Model file for the job. Use its own axes, mm. A direction names the side the tool comes from. Give positions to 0.01 mm unless a question says otherwise; leave off trailing zeros. Write each loop counter-clockwise with the first axis right and the second up, starting at its lowest first coordinate (ties: lowest second). Pieces come first, ordered by that corner, then holes. Notation, with made-up numbers: M 75,48.5 L 131,48.5 A18 cw 131,71.5 Z; hole C -15.75,15.25 d5. An arc over 180 degrees is marked long. Answer as a JSON object with one key per item and string values. Group by question number.
```python
from build123d import *

# Parameters (mm, degrees)
SKETCH_1_W          = 15
SKETCH_1_H          = 15
EXTRUDE_1_DEPTH     = 100
SKETCH_2_W          = 45
SKETCH_2_H          = 15
EXTRUDE_2_DEPTH     = 10
SKETCH_3_R          = 2.5
CUT_EXTRUDE_1_DEPTH = 20
SKETCH_5_W          = 45
SKETCH_5_H          = 19.472765692
EXTRUDE_3_DEPTH     = 10
SKETCH_6_R          = 2.5
CUT_EXTRUDE_2_DEPTH = 103.961386699


with BuildPart() as part:
    # 草图1 → 凸台-拉伸1 (new body)
    with BuildSketch(Plane.XY):
        Rectangle(SKETCH_1_W, SKETCH_1_H)
    extrude(amount=EXTRUDE_1_DEPTH)

    # 草图2 → 凸台-拉伸2 (add)
    with BuildSketch(Plane.XY.offset(100)):
        Rectangle(SKETCH_2_W, SKETCH_2_H)
    extrude(amount=-EXTRUDE_2_DEPTH)

    # 草图3 → 切除-拉伸1 (cut)
    with BuildSketch(Plane.XY.offset(100)):
        with Locations((-16.5, 0)):
            Circle(SKETCH_3_R)
        with Locations((16.5, 0)):
            Circle(SKETCH_3_R)
    extrude(amount=-CUT_EXTRUDE_1_DEPTH, mode=Mode.SUBTRACT)

    # 草图5 → 凸台-拉伸3 (add)
    with BuildSketch(Plane(origin=(0, 0, 0), x_dir=(-1, 0, 0), z_dir=(0, 0, -1))):
        Rectangle(SKETCH_5_W, SKETCH_5_H)
    extrude(amount=-EXTRUDE_3_DEPTH)

    # 草图6 → 切除-拉伸2 (cut, through all)
    with BuildSketch(Plane(origin=(0, 0, 0), x_dir=(-1, 0, 0), z_dir=(0, 0, -1))):
        with Locations(Location((-16.5, 0, 0), (0, 0, 180))):
            Circle(SKETCH_6_R)
        with Locations(Location((16.5, 0, 0), (0, 0, 180))):
            Circle(SKETCH_6_R)
    extrude(amount=-CUT_EXTRUDE_2_DEPTH, mode=Mode.SUBTRACT)


solid = part.part
```
Q1. Slice it at B-B, the plane x = 16.5. Write the cut outline in (y, z).
Q2. Slice it at D-D, the plane y = -6.25. Write the cut outline in (x, z).
Q3. 3-axis set-ups, long thin cutter, end or side, ignore diameter. For faces 4 (the flat face through (7.5, 0, 49)), 5 (the flat face through (0, -7.5, 66)), 6 (the flat face through (-13, 0, 90)), 7 (the flat face through (0, 7.5, 66)): which of +Z, -Z, +X, -X, +Y, -Y reach the whole face in a straight line?
Q4. Slice it at A-A, the plane y = 1.5. Write the cut outline in (x, z).
Q5. Drop flat-ended pins along their axis: P1, Ø2, axis at x = -6.5, z = 68.5, coming from the -Y side; P2, Ø5, axis at y = -2, z = 51, coming from the -X side; P3, Ø3, axis at x = 4.5, z = 45.5, coming from the +Y side. Give the stop position or say it passes through.
Q6. Slice it at C-C, the plane x = 4. Write the cut outline in (y, z).
Q7. Two-plate mould, pull along Z, no slides. Class faces 1 (the flat face through (0, 0, 100)), 2 (the flat face through (0, 9, 10)), 3 (the cylindrical face through (14, 0, 5)): +Z half, -Z half, draft (parallel to the pull), parting line (faces both ways), or undercut.
Q8. Wall check: L1, parallel to Y at x = -16.5, z = 96.25; L2, parallel to Z at x = -14, y = -0.75; L3, parallel to Y at x = -16.5, z = 8. Give the ranges that are in metal, low to high.
Solved:
{
 "1": {"outline": "M -9.74,0 L -2.5,0 L -2.5,10 L -9.74,10 Z; M -7.5,90 L -2.5,90 L -2.5,100 L -7.5,100 Z; M 2.5,0 L 9.74,0 L 9.74,10 L 2.5,10 Z; M 2.5,90 L 7.5,90 L 7.5,100 L 2.5,100 Z"},
 "2": {"outline": "M -22.5,0 L 22.5,0 L 22.5,10 L 7.5,10 L 7.5,90 L 22.5,90 L 22.5,100 L -22.5,100 L -22.5,90 L -7.5,90 L -7.5,10 L -22.5,10 Z"},
 "3": {"face 4": "+X, +Y, -Y", "face 5": "+Z, +X, -X, -Y", "face 6": "-X, +Y, -Y", "face 7": "+Z, +X, -X, +Y"},
 "4": {"outline": "M -22.5,0 L -18.5,0 L -18.5,10 L -22.5,10 Z; M -22.5,90 L -18.5,90 L -18.5,100 L -22.5,100 Z; M -14.5,0 L 14.5,0 L 14.5,10 L 7.5,10 L 7.5,90 L 14.5,90 L 14.5,100 L -14.5,100 L -14.5,90 L -7.5,90 L -7.5,10 L -14.5,10 Z; M 18.5,0 L 22.5,0 L 22.5,10 L 18.5,10 Z; M 18.5,90 L 22.5,90 L 22.5,100 L 18.5,100 Z"},
 "5": {"P1": "stops at y = -7.5", "P2": "stops at x = -7.5", "P3": "stops at y = 7.5"},
 "6": {"outline": "M -9.74,0 L 9.74,0 L 9.74,10 L 7.5,10 L 7.5,100 L -7.5,100 L -7.5,10 L -9.74,10 Z"},
 "7": {"face 1": "+Z half", "face 2": "undercut", "face 3": "draft"},
 "8": {"L1": "y = -7.5 to -2.5, 2.5 to 7.5", "L2": "z = 0 to 10, 90 to 100", "L3": "y = -9.74 to -2.5, 2.5 to 9.74"}
}
